For this review, take the finished solid that the model builds, in its own axes (mm). Give positions to 0.01 mm unless a question says otherwise; leave off trailing zeros. Use CSV: the item, a comma, the result in double quotes. Start each with the question number.
1. For pin 1 (0.9 mm diameter, centred on y = 2, z = 163, fed in from -X); pin 2 (0.9 mm diameter, centred on x = -196.5, y = 1.5, fed in from +Z); pin 3 (4.5 mm diameter, centred on x = -160, z = 124, fed in from +Y); pin 4 (1.5 mm diameter, centred on x = -177.5, y = 1.5, fed in from -Z), all flat-tipped, find the tip position at first contact; note any pin that passes through.
2. Wall thickness on line 1 (Z direction, x = 160, y = 0.75); line 2 (Z direction, x = -206.5, y = 1.85); line 3 (X direction, y = 1.5, z = 160): over which ranges is each line inside the solid? List them lowest first.
3. Take a section at A-A on y = 0.8. State how many separate pieces and enclosed holes the cut face has, plus the area to 3 significant figures.
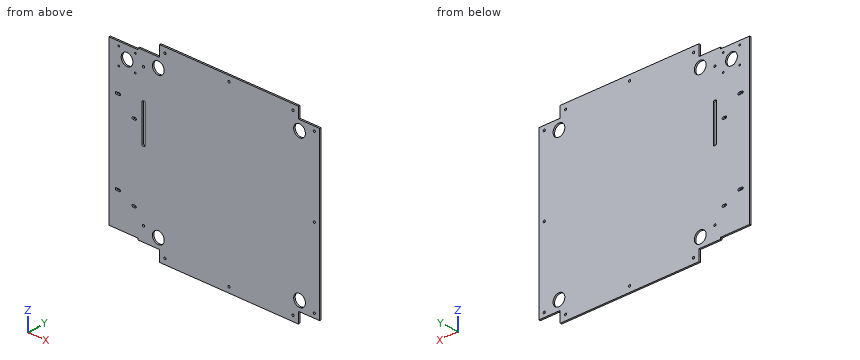
```python
from build123d import *

# Parameters (mm, degrees)
SKETCH1_8_R         = 11
SKETCH1_8_R_2       = 2
SKETCH1_8_R_3       = 1.5
BOSS_EXTRUDE5_DEPTH = 3


with BuildPart() as part:
    # Sketch1_8 → Boss-Extrude5 (new body)
    with BuildSketch(Plane(origin=(0, 0, 0), x_dir=(1, 0, 0), z_dir=(0, 1, 0))):
        Polygon((130, -150), (170, -150), (170, 150), (130, 150), (130, 170), (-130, 170), (-130, 150), (-170, 150), (-170, 147), (-225, 147), (-225, -147), (-170, -147), (-170, -150), (-130, -150), (-130, -170), (130, -170), align=None)
        with Locations(Location((-132.375, 132.375, 0), (0, 0, 270))):
            Circle(SKETCH1_8_R, mode=Mode.SUBTRACT)
        with Locations(Location((132.375, 132.375, 0), (0, 0, 270))):
            Circle(SKETCH1_8_R, mode=Mode.SUBTRACT)
        with Locations(Location((-132.375, -132.375, 0), (0, 0, 270))):
            Circle(SKETCH1_8_R, mode=Mode.SUBTRACT)
        with Locations(Location((132.375, -132.375, 0), (0, 0, 270))):
            Circle(SKETCH1_8_R, mode=Mode.SUBTRACT)
        with Locations(Location((160, -142, 0), (0, 0, 270))):
            Circle(SKETCH1_8_R_2, mode=Mode.SUBTRACT)
        with Locations(Location((160, 0, 0), (0, 0, 270))):
            Circle(SKETCH1_8_R_2, mode=Mode.SUBTRACT)
        with Locations(Location((160, 142, 0), (0, 0, 270))):
            Circle(SKETCH1_8_R_2, mode=Mode.SUBTRACT)
        with Locations(Location((120, -160, 0), (0, 0, 270))):
            Circle(SKETCH1_8_R_2, mode=Mode.SUBTRACT)
        with Locations(Location((-120, -160, 0), (0, 0, 270))):
            Circle(SKETCH1_8_R_2, mode=Mode.SUBTRACT)
        with Locations(Location((0, -160, 0), (0, 0, 270))):
            Circle(SKETCH1_8_R_2, mode=Mode.SUBTRACT)
        with Locations(Location((120, 160, 0), (0, 0, 270))):
            Circle(SKETCH1_8_R_2, mode=Mode.SUBTRACT)
        with Locations(Location((-120, 160, 0), (0, 0, 270))):
            Circle(SKETCH1_8_R_2, mode=Mode.SUBTRACT)
        with Locations(Location((0, 160, 0), (0, 0, 270))):
            Circle(SKETCH1_8_R_2, mode=Mode.SUBTRACT)
        with BuildLine():
            ThreePointArc((-157, -68.911348687), (-157.585786438, -70.325562249), (-159, -70.911348687))
            Line((-159, -70.911348687), (-161, -70.911348687))
            ThreePointArc((-161, -70.911348687), (-162.414213562, -70.325562249), (-163, -68.911348687))
            Line((-163, -68.911348687), (-163, -2))
            ThreePointArc((-163, -2), (-162.414213562, -0.585786438), (-161, 0))
            Line((-161, 0), (-159, 0))
            ThreePointArc((-159, 0), (-157.585786438, -0.585786438), (-157, -2))
            Line((-157, -2), (-157, -68.911348687))
        make_face(mode=Mode.SUBTRACT)
        with Locations(Location((-160, 124, 0), (0, 0, 270))):
            Circle(SKETCH1_8_R_2, mode=Mode.SUBTRACT)
        with Locations(Location((-160, -124, 0), (0, 0, 270))):
            Circle(SKETCH1_8_R_2, mode=Mode.SUBTRACT)
        with Locations(Location((-175.5, -108.5, 0), (0, 0, 270))):
            Circle(SKETCH1_8_R_3, mode=Mode.SUBTRACT)
        with Locations(Location((-206.5, -139.5, 0), (0, 0, 270))):
            Circle(SKETCH1_8_R_3, mode=Mode.SUBTRACT)
        with Locations(Location((-175.5, -139.5, 0), (0, 0, 270))):
            Circle(SKETCH1_8_R_3, mode=Mode.SUBTRACT)
        with Locations(Location((-191, -124, 0), (0, 0, 270))):
            Circle(SKETCH1_8_R, mode=Mode.SUBTRACT)
        with Locations(Location((-206.5, -108.5, 0), (0, 0, 270))):
            Circle(SKETCH1_8_R_3, mode=Mode.SUBTRACT)
        with BuildLine():
            ThreePointArc((-211.1, -66.5), (-213.1, -64.5), (-211.1, -62.5))
            Line((-211.1, -62.5), (-205.1, -62.5))
            ThreePointArc((-205.1, -62.5), (-203.1, -64.5), (-205.1, -66.5))
            Line((-205.1, -66.5), (-211.1, -66.5))
        make_face(mode=Mode.SUBTRACT)
        with BuildLine():
            ThreePointArc((-179.6, -39), (-181.6, -37), (-179.6, -35))
            Line((-179.6, -35), (-175.6, -35))
            ThreePointArc((-175.6, -35), (-173.6, -37), (-175.6, -39))
            Line((-175.6, -39), (-179.6, -39))
        make_face(mode=Mode.SUBTRACT)
        with BuildLine():
            ThreePointArc((-211.1, 83.4), (-213.1, 85.4), (-211.1, 87.4))
            Line((-211.1, 87.4), (-205.1, 87.4))
            ThreePointArc((-205.1, 87.4), (-203.1, 85.4), (-205.1, 83.4))
            Line((-205.1, 83.4), (-211.1, 83.4))
        make_face(mode=Mode.SUBTRACT)
        with BuildLine():
            ThreePointArc((-179.6, 98), (-181.6, 100), (-179.6, 102))
            Line((-179.6, 102), (-175.6, 102))
            ThreePointArc((-175.6, 102), (-173.6, 100), (-175.6, 98))
            Line((-175.6, 98), (-179.6, 98))
        make_face(mode=Mode.SUBTRACT)
    extrude(amount=BOSS_EXTRUDE5_DEPTH)


solid = part.part
```
Check result:
1,pin 1,"stops at x = -130"
1,pin 2,"stops at z = 147"
1,pin 3,"stops at y = 3"
1,pin 4,"stops at z = -147"
2,line 1,"z = -150 to -144, -140 to -2, 2 to 140, 144 to 150"
2,line 2,"z = -147 to -87.4, -83.4 to 62.5, 66.5 to 107, 110 to 138, 141 to 147"
2,line 3,"x = -130 to -122, -118 to -2, 2 to 118, 122 to 130"
3,separate pieces,"1"
3,enclosed holes,"25"
3,area,"126,000 mm²"
